CAD build for the part. Positions are in the model's coordinates, mm. A direction names the side the tool comes from. Give positions to 0.01 mm unless a question says otherwise; leave off trailing zeros. Loops run counter-clockwise (first coordinate to the right, second up) from the corner with the lowest first, then second, coordinate; pieces in that order, holes last.
Item 1: Which spindle directions (+Z, -Z, +X, -X, +Y, -Y) get a long thin tool onto all of the face, cutting with end or side? Do faces 4 (the cylindrical face through (-3.806, 1.984, 1.438)), 5 (the flat face through (-1.1, 0, 1.3)), 6 (the flat face through (0, 7, -3)). Say none if no direction does.
Item 2: Saw through at B-B on y = -0.5. Give the cut face in (x, z).
Item 3: Saw through at C-C on z = 4.25. Give the number of separate pieces and of enclosed holes in the cut face, plus the area to 3 significant figures.
Item 4: Saw through at A-A on y = 2.75. Give the cut face in (x, z), plus the area to 3 significant figures.
Item 5: Mould opens along Y. For faces 1 (the flat face through (0, -3, -2.2)), 2 (the cylindrical face through (-4.515, -3.444, 0.436)), 3 (the conical face through (0.1, -7.17, 2.72)) say: released by +Y, released by -Y, zero draft, split by the parting line, or undercut.
Item 6: Saw through at D-D on y = -6. Give the cut face in (x, z).
Item 7: Drop flat-ended pins along their axis: P1, Ø1, axis at x = -3, y = -3, coming from the +Z side; P2, Ø4, axis at y = -5, z = 4, coming from the +X side; P3, Ø4, axis at x = 1, z = -0.5, coming from the -Y side; P4, Ø4.5, axis at y = -4.83, z = 0, coming from the -X side. Give the stop position or say it passes through.
Item 8: Probe probe 1 along X at (y, z) = (-6.5, 0); probe 2 along X at (y, z) = (4.7, 0); probe 3 along Y at (x, z) = (2.75, -5.75). List the from-to ranges inside material, lowest first.
Autodesk Inventor part; units mm, degrees
ref_plane "YZ Plane" through (0, 0, 0) normal (1, 0, 0) x (0, 1, 0)
ref_plane "XZ Plane" through (0, 0, 0) normal (0, 1, 0) x (-1, 0, 0)
ref_plane "XY Plane" through (0, 0, 0) normal (0, 0, 1) x (1, 0, 0)
sketch "Sketch1" plane through (0, 0, 0) normal (0, 1, 0) x (-1, 0, 0)
  circle A0 centre (0, 0) radius 7
  line L0 (0, -9.8) -> (0, 9.8) construction
  circle A1 centre (0, 0) radius 1.4
  dimension "d0" = 14
  dimension "d42" = 2.8
extrude "Extrusion1" add sketch "Sketch1" along normal blind 7
sketch "Sketch2" plane through (0, 0, 0) normal (0, -1, 0) x (1, 0, 0)
  circle A0 centre (0, 0) radius 1.45
  arc A1 (1.2894, -2.2) -> (-1.2894, -2.2) centre (0, 0) ccw
  line L0 (-1.2894, -2.2) -> (1.2894, -2.2)
  circle A2 centre (0, 0) radius 7
  dimension "d4" = 5.1
  dimension "d5" = 2.2
extrude "Extrusion2" add sketch "Sketch2" along normal blind 8 contours A2
ref_plane "Work Plane1" through (0, 6, 0) normal (0, -1, 0) x (1, 0, 0)
sketch "Sketch5" plane through (0, 0, 0) normal (1, 0, 0) x (0, 1, 0)
  line L0 (0, 7) -> (7, 7)
  line L1 (4.6942, 7) -> (5.9942, 7)
  line L2 (5.9942, 7) -> (5.9942, 5)
  line L3 (5.9942, 5) -> (4.6942, 5)
  line L4 (4.6942, 5) -> (4.6942, 7)
  point P0 (0, 0)
  dimension "d17" = 1.3
  dimension "d18" = 2
sketch "Sketch6" plane through (0, 0, 0) normal (1, 0, 0) x (0, 1, 0)
  circle A0 centre (2.1729, 0) radius 1.45
  line L0 (-8, -7) -> (7, -7)
  point P0 (0, 0)
  dimension "d43" = 2.9
  dimension "d44" = 7
extrude "Extrusion5" cut sketch "Sketch6" against normal blind 10
pattern_circular "Circular Pattern3" count 3 over 360 about axis through (0, 0, 0) along (0, 1, 0) of "Extrusion5"
chamfer "Chamfer4" distance 1 angle 45 3 edges at (1.4, 7, 0) (0, -8, 2.55) (0, -8, -2.2)
pattern_linear "Rectangular Pattern2" count 2 spacing 7 along (0, -1, 0) of "Extrusion5", "Circular Pattern3"
properties part number "00_Motorcoupling_5mm_M3"
Results below:
1. face 4: -X
1. face 5: -Y
1. face 6: +Z, -Z, +X, -X, +Y
2. outline: circle Ø14 at (0, 0); hole (-1.29, -2.2) - (1.29, -2.2) arc R2.55 ccw (long way) to start
3. separate pieces: 1
3. enclosed holes: 2
3. area: 152 mm2
4. outline: (-6.87, -1.33) arc R7 ccw to (2.28, -6.62) - (-0.77, -1.33) - close; (-6.87, 1.33) - (-0.77, 1.33) - (2.28, 6.62) arc R7 ccw to start; (1.54, 0) - (4.59, -5.29) arc R7 ccw to (4.59, 5.29) - close
4. area: 101 mm2
5. face 1: zero draft
5. face 2: undercut
5. face 3: released by -Y
6. outline: (-6.95, -0.85) arc R7 ccw to (2.74, -6.44) - (0.29, -2.2) - (-1.29, -2.2) arc R2.55 cw to (-2.4, -0.85) - close; (-6.95, 0.85) - (-2.4, 0.85) arc R2.55 cw to (0.46, 2.51) - (2.74, 6.44) arc R7 ccw to start; (1.94, -1.66) - (4.21, -5.59) arc R7 ccw to (4.21, 5.59) - (1.94, 1.66) arc R2.55 cw to start
7. P1: stops at z = 6.54
7. P2: stops at x = 6.71
7. P3: stops at y = -7.57
7. P4: stops at x = -7
8. probe 1: x = -7 to -2.55, 2.55 to 7
8. probe 2: x = -7 to -1.4, 1.4 to 7
8. probe 3: y = -8 to -6.19, -3.46 to 0.81, 3.54 to 7
